from build123d import *

# Parameters (mm, degrees)
F0_W     = 98.692965
F0_H     = 101.042532
F1_DEPTH = 100
F2_R     = 10
F3_T     = -5


with BuildPart() as f1:
    # F0 (on Top) → F1 (new body)
    with BuildSketch(Plane.XY):
        with Locations((-14.294499, -1.221735)):
            Rectangle(F0_W, F0_H)
    extrude(amount=F1_DEPTH)

    # F2
    f2_edges = [f1.edges().sort_by_distance(p)[0] for p in [
        (-14.2945, -51.743001, 100),
        (35.051983, -1.221735, 100),
        (-14.2945, 49.299531, 100),
        (-63.640982, -1.221735, 100),
    ]]
    fillet(f2_edges, radius=F2_R)

    # F3
    f3_openings = [f1.faces().sort_by_distance(p)[0] for p in [
        (-14.2945, -1.221735, 0),
    ]]
    offset(amount=F3_T, openings=f3_openings)


solid = f1.part
Design review of the part built by this model. Coordinates are the model's own, in mm. A direction names the side the tool comes from. Give positions to 0.01 mm unless a question says otherwise; leave off trailing zeros. Loops run counter-clockwise (first coordinate to the right, second up) from the corner with the lowest first, then second, coordinate; pieces in that order, holes last. Notation, with made-up numbers: (18, 65.5) - (47, 65.5) arc R24 cw to (47, 77.5) - close; hole circle Ø9 at (-15, 67). An arc over 180 degrees is marked (long way). Use CSV: the item, a comma, the result in double quotes. Start each with the question number.
1. Add section B-B (x = -25.5). State the section outline as (y, z) points, plus the area to 3 significant figures.
2. Machinability: for faces 4 (the cylindrical face through (28.626, -0.584, 93.496)), 5 (the cylindrical face through (-13.604, -48.891, 96.993)), which of the approach directions +Z, -Z, +X, -X, +Y, -Y give a long, thin tool a straight path to every point of the face, cutting with its end or side? Answer none if there is none.
3. Add section D-D (z = 93.5). State the section outline as (x, y) points.
4. Wall thickness on L1, parallel to Y at x = -35, z = 48.5; L2, parallel to X at y = -14.5, z = 52; L3, parallel to Z at x = -25.5, y = -37.5: over which ranges is each line inside the solid? List them lowest first.
5. Add section A-A (z = 7.5). State the section outline as (x, y) points.
6. Draft analysis for pull direction X (two halves, no side actions). For faces 1 (the cylindrical face through (-13.674, -45.317, 93.496)), 2 (the flat face through (-15, -1, 100)), 3 (the cylindrical face through (-60.79, -0.51, 96.99)), state which applies: released by +X, released by -X, zero draft, split by the parting line, or undercut.
7. Add section C-C (y = 11). State the section outline as (x, z) points, plus the area to 3 significant figures.
8. Insertion check: P1, Ø10, axis at x = -0.5, y = 13.5, coming from the -Z side. The pin has a flat end and moves straight along its axis. Give the tip position at first contact, or say it passes through.
Results found:
1,outline,"(-51.74, 0) - (-46.74, 0) - (-46.74, 90) arc R5 cw to (-41.74, 95) - (39.3, 95) arc R5 cw to (44.3, 90) - (44.3, 0) - (49.3, 0) - (49.3, 90) arc R10 ccw to (39.3, 100) - (-41.74, 100) arc R10 ccw to (-51.74, 90) - close"
1,area,"1,420 mm²"
2,face 4,"-Z"
2,face 5,"+Z, +X, -X, -Y"
3,outline,"(-63.01, -51.11) - (34.42, -51.11) - (34.42, 48.67) - (-63.01, 48.67) - close; hole (-57.21, -45.31) - (28.62, -45.31) - (28.62, 42.87) - (-57.21, 42.87) - close"
4,L1,"y = -51.74 to -46.74, 44.3 to 49.3"
4,L2,"x = -63.64 to -58.64, 30.05 to 35.05"
4,L3,"z = 95 to 100"
5,outline,"(-63.64, -51.74) - (35.05, -51.74) - (35.05, 49.3) - (-63.64, 49.3) - close; hole (-58.64, -46.74) - (30.05, -46.74) - (30.05, 44.3) - (-58.64, 44.3) - close"
6,face 1,"undercut"
6,face 2,"zero draft"
6,face 3,"released by -X"
7,outline,"(-63.64, 0) - (-58.64, 0) - (-58.64, 90) arc R5 cw to (-53.64, 95) - (25.05, 95) arc R5 cw to (30.05, 90) - (30.05, 0) - (35.05, 0) - (35.05, 90) arc R10 ccw to (25.05, 100) - (-53.64, 100) arc R10 ccw to (-63.64, 90) - close"
7,area,"1,410 mm²"
8,P1,"stops at z = 95"
